Design review of the part shown in the three views and the two pictorial views. Dimensions are in mm from the part's minimum x, y and z. Coordinates: 2 decimals unless noted, no trailing zeros. Loops run counter-clockwise (first coordinate to the right, second up) from the corner with the lowest first, then second, coordinate; pieces in that order, holes last. Notation, with made-up numbers: (47.25, -18.5) -> (81.25, -18.5) arc R28 cw to (81.25, 1.5) -> close; hole circle Ø7 at (61.5, 39). An arc over 180 degrees is marked (long way). One line per item, written item: value. Start each with the question number.
1. Add section B-B on y = 10.25. Give the number of separate pieces and of enclosed holes in the cut face, plus the area to 3 significant figures.
2. Add section C-C on x = 374.65. Write out the cut boundary in (y, z).
3. Add section A-A on x = 316.23. Write out the cut boundary in (y, z), plus the area to 3 significant figures.
4. Insertion check: pin 1 (12.5 mm diameter, centred on x = 50.8, z = 19.05, fed in from +Y); pin 2 (5.5 mm diameter, centred on x = 99.06, z = 19.05, fed in from -Y); pin 3 (6.5 mm diameter, centred on x = 152, y = 8.5, fed in from -Z); pin 4 (4 mm diameter, centred on x = 115.5, y = 8, fed in from +Z). Each pin has a flat end and moves straight along its axis. Give the tip position at first contact, or say it passes through.
5. For probe 1 along Z at (x, y) = (50.8, 4.5); probe 2 along X at (y, z) = (3, 30); probe 3 along X at (y, z) = (9.75, 28), list the stretches that pass through material, from the lowest coordinate up.
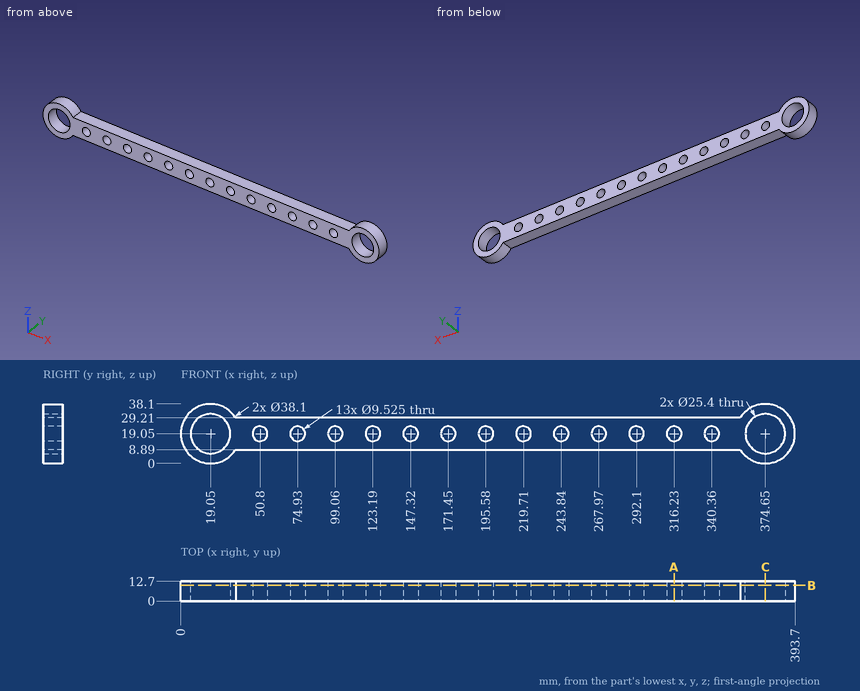
Worked answers:
1. separate pieces: 1
1. enclosed holes: 15
1. area: 6,830 mm²
2. outline: (0, 0) -> (12.7, 0) -> (12.7, 6.35) -> (0, 6.35) -> close; (0, 31.75) -> (12.7, 31.75) -> (12.7, 38.1) -> (0, 38.1) -> close
3. outline: (0, 8.89) -> (12.7, 8.89) -> (12.7, 14.29) -> (0, 14.29) -> close; (0, 23.81) -> (12.7, 23.81) -> (12.7, 29.21) -> (0, 29.21) -> close
3. area: 137 mm²
4. pin 1: stops at y = 12.7
4. pin 2: passes through
4. pin 3: stops at z = 8.89
4. pin 4: stops at z = 29.21
5. probe 1: z = 8.89 to 14.29, 23.81 to 29.21
5. probe 2: x = 3.46 to 12.62, 25.48 to 34.64, 359.06 to 368.22, 381.08 to 390.24
5. probe 3: x = 2.23 to 10.04, 28.06 to 365.64, 383.66 to 391.47
